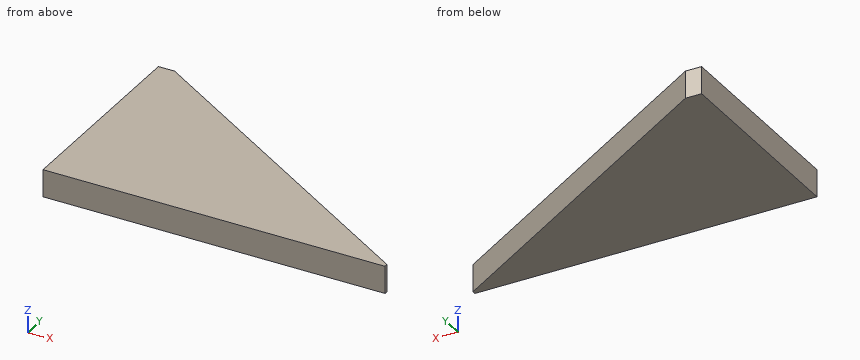
```python
from build123d import *

# Parameters (mm, degrees)
ESQUISSE1_W             = 8
ESQUISSE1_H             = 60
BOSS_EXTRU_1_DEPTH      = 100
ENL_V_MAT_EXTRU_1_REACH = 10


with BuildPart() as part:
    # Esquisse1 → Boss.-Extru.1 (new body)
    with BuildSketch(Plane(origin=(0, 0, 0), x_dir=(0, 0, -1), z_dir=(1, 0, 0))):
        with Locations((-0.854369973, 29.104551848)):
            Rectangle(ESQUISSE1_W, ESQUISSE1_H)
    extrude(amount=-BOSS_EXTRU_1_DEPTH)

    # Esquisse2 → Enlèv. mat.-Extru.1 (cut, up to next)
    with BuildSketch(Plane.XY.offset(4.854369973), mode=Mode.PRIVATE) as enl_v_mat_extru_1_sk1:
        Polygon((-96, 59.563838708), (1.070476381, 60.732011114), (2.184337253, -1.224933167), align=None)
    enl_v_mat_extru_1_tool1 = extrude(enl_v_mat_extru_1_sk1.sketch, amount=-ENL_V_MAT_EXTRU_1_REACH, mode=Mode.PRIVATE) & part.part
    add(enl_v_mat_extru_1_tool1.solids().sort_by_distance((-30.915062, 39.690306, 4.85437))[0], mode=Mode.SUBTRACT)


solid = part.part
```
Geometry check sheet. Reference: the model listing, model coordinates, mm. Round coordinates to 2 decimals unless told otherwise and drop trailing zeros. Loops run counter-clockwise (first coordinate to the right, second up) from the corner with the lowest first, then second, coordinate; pieces in that order, holes last. Notation, with made-up numbers: (15, -10.75) - (25, -10.75) arc R15 ccw to (25, 1.25) - close; hole circle Ø1 at (42, -3). An arc over 180 degrees is marked (long way). Write item = value, one per line. Start each with the question number.
1. Section check B-B on x = -17.5. Enter the section's corners in (y, z).
2. Thickness scan on line 1 (Y direction, x = -79, z = 1); line 2 (X direction, y = 56.5, z = -2.5); line 3 (Y direction, x = -30.5, z = 2). Record the ranges inside material, lowest first.
3. Section check C-C on y = 55.5. Enter the section's corners in (x, z).
4. Depth check by flat-ended pin: pin 1 (4 mm diameter, centred on y = 48.5, z = 2, fed in from +X); pin 2 (1.5 mm diameter, centred on x = -46, z = 3.5, fed in from +Y). Enter the tip coordinate at first touch or a pass-through.
5. Section check A-A on z = -0.25. Enter the section's corners in (x, y), then the cut area to 3 significant figures.
Working result:
q1.outline = (-0.9, -3.15) - (10.96, -3.15) - (10.96, 4.85) - (-0.9, 4.85) - close
q2.line_1 = -0.9 to 49.04
q2.line_2 = -100 to -91.05
q2.line_3 = -0.9 to 19.01
q3.outline = (-100, -3.15) - (-89.44, -3.15) - (-89.44, 4.85) - (-100, 4.85) - close
q4.pin_1 = -74.9
q4.pin_2 = 29.07
q5.outline = (-100, -0.9) - (0, -0.9) - (0, 0.13) - (-95.26, 59.1) - (-100, 59.1) - close
q5.area = 3,190 mm^2
